```python
from build123d import *

# Parameters (mm, degrees)
SKETCH1_R           = 1.5
BOSS_EXTRUDE1_DEPTH = 7.5
FILLET1_R           = 2.54
CHAMFER2_SIZE       = 2.665692085
CHAMFER2_SIZE_2     = 5
SKETCH4_R           = 1.75
BOSS_EXTRUDE2_DEPTH = 1.5
FILLET2_R           = 1.500000048
CUT_EXTRUDE1_DEPTH  = 7.5


# Some blends are built 0.0001 mm under size
with BuildPart() as part:
    # Sketch1 → Boss-Extrude1 (new body)
    with BuildSketch(Plane.XY):
        with BuildLine():
            Line((17.881226168, -7.264400992), (12.820526555, -5.392684832))
            ThreePointArc((12.820526555, -5.392684832), (10.249738142, -3.113969145), (7.665252761, -5.377138064))
            Line((7.665252761, -5.377138064), (-11.113294597, -4.678112359))
            Line((-11.113294597, -4.678112359), (-11.797383791, -5.362201553))
            Line((-11.797383791, -5.362201553), (-11.797383791, -6.482688956))
            Line((-11.797383791, -6.482688956), (6.932172042, -7.212884314))
            Line((6.932172042, -7.212884314), (8.80911881, -7.87994093))
            ThreePointArc((8.80911881, -7.87994093), (9.985840847, -8.298026499), (11.221708583, -8.118858325))
            Line((11.221708583, -8.118858325), (13.521910205, -7.18234795))
            Line((13.521910205, -7.18234795), (20.245554573, -9.191065966))
            Line((20.245554573, -9.191065966), (20.849339495, -6.668640767))
            Line((20.849339495, -6.668640767), (19.081317898, -5.499046666))
            Line((19.081317898, -5.499046666), (18.665024161, -5.64566597))
            Line((18.665024161, -5.64566597), (18.356685028, -6.933810758))
            Line((18.356685028, -6.933810758), (17.881226168, -7.264400992))
        make_face()
        with Locations((10.241902304, -5.712315853)):
            Circle(SKETCH1_R, mode=Mode.SUBTRACT)
    extrude(amount=BOSS_EXTRUDE1_DEPTH)

    # Fillet1
    fillet1_edges = [part.edges().sort_by_distance(p)[0] for p in [
        (13.521910205, -7.18234795, 3.75),
    ]]
    fillet(fillet1_edges, radius=FILLET1_R)

    # Chamfer2
    # the kernel refuses this chamfer: 5, 2.665692085 mm, written as the material it takes off along each edge
    with BuildSketch(Plane(origin=(-11.113294597, -4.678112359, -12.981362455), x_dir=(-0.7323937898878367, -0.6808812940107337, 0), z_dir=(0, 0, 1))) as chamfer2_piece_1:
        Polygon((CHAMFER2_SIZE * 0.999336395545, CHAMFER2_SIZE * 0.0364248351519), (-CHAMFER2_SIZE_2 * 0.706558829098, CHAMFER2_SIZE_2 * 0.707654308984), (0, 0), align=None)
    extrude(amount=33.462724911, mode=Mode.SUBTRACT)

    # Sketch4 → Boss-Extrude2 (add)
    with BuildSketch(Plane(origin=(-0.189278476, -5.084755532, 0), x_dir=(0.9993078802351368, -0.03719893143569399, 0), z_dir=(0.03719893143569399, 0.9993078802351368, 0))):
        with Locations((0.885514773, -3.75)):
            Circle(SKETCH4_R)
    extrude(amount=BOSS_EXTRUDE2_DEPTH)

    # Fillet2
    fillet2_edges = [part.edges().sort_by_distance(p)[0] for p in [
        (-0.997366978, -3.553635785, 3.75),
    ]]
    fillet(fillet2_edges, radius=FILLET2_R - 0.0001)  # a hair under: the kernel refuses the full size

    # Sketch5 → Cut-Extrude1 (cut)
    with BuildSketch(Plane.XY.offset(7.5)):
        Polygon((20.405496385, -6.375026546), (19.765742241, -9.047719944), (20.245554573, -9.191065966), (20.849339495, -6.668640767), align=None)
    extrude(amount=-CUT_EXTRUDE1_DEPTH, mode=Mode.SUBTRACT)


solid = part.part
```
Design review of the part built by this model. Coordinates are the model's own, in mm. A direction names the side the tool comes from. Give positions to 0.01 mm unless a question says otherwise; leave off trailing zeros. Order: outer loops, then holes, each group sorted by start corner. A loop starts at its lowest first (then second) coordinate and runs counter-clockwise, first axis right, second up. Notation, with made-up numbers: M 74,74.5 L 99,74.5 A17 cw 99,78.5 Z; hole C -13,13 d2. An arc over 180 degrees is marked long. One line per question, with ' | ' between items. Start each with the question number.
Q1. For L1, parallel to X at y = -4.55, z = 5.25; L2, parallel to Y at x = 4, z = 4.5; L3, parallel to Y at x = 8, z = 2.5, list the stretches that pass through material, from the lowest coordinate up. Write a range as [from, to].
Q2. We need section B-B (x = 6). Write out the cut boundary in (y, z).
Q3. For pin 1 Ø1 at (x, z) = (2, 3) entering from -Y, flat-tipped, find the tip position at first contact; note if it passes through.
Q4. We need section C-C (x = 14). Write out the cut boundary in (y, z).
Q5. The part is to be moulded in two halves that separate along X. For faces 4 (the face through (7.858, -7.542, 3.698)), 5 (the face through (5, -6, 0)), 6 (the face through (11.947, -7.823, 3.698)), 7 (the face through (17.03, -8.23, 3.7)), say which applies: +X half, -X half, draft (parallel to the pull), parting line (faces both ways), or undercut.
Q6. Machinability: for faces 1 (the face through (20.09, -7.69, 3.8)), 2 (the face through (2.4, -5.18, 2.86)), 3 (the face through (15.386, -6.342, 3.698)), which of the approach directions +Z, -Z, +X, -X, +Y, -Y give a long, thin tool a straight path to every point of the face, cutting with its end or side? Answer none if there is none.
Q7. We need section A-A (z = 0.75). Write out the cut boundary in (x, y), plus the area to 3 significant figures.
Returned:
1) L1: [0.03, 1.35], [7.92, 9.29], [11.19, 12.57] | L2: [-7.1, -5.24] | L3: [-7.59, -4.4]
2) outline: M -7.18,0 L -5.32,0 L -5.32,7.5 L -7.18,7.5 Z
3) pin 1: y = -7.04
4) outline: M -7.36,0 L -5.83,0 L -5.83,7.5 L -7.36,7.5 Z
5) face 4: -X half | face 5: draft | face 6: undercut | face 7: undercut
6) face 1: +Z, -Z, +X, -Y | face 2: +Y | face 3: +Z, -Z, +Y
7) outline: M -11.8,-6.48 L 6.93,-7.21 L 8.81,-7.88 A2.6 ccw 11.22,-8.12 L 12.69,-7.52 A2.54 cw 14.38,-7.44 L 19.77,-9.05 L 20.41,-6.38 L 19.08,-5.5 L 18.67,-5.65 L 18.36,-6.93 L 17.88,-7.26 L 12.82,-5.39 A2.6 ccw 7.67,-5.38 L -6.12,-4.86 L -11.8,-6.27 Z; hole C 10.24,-5.71 d3 | area: 59.9 mm2
